Work out the finished part from the listing and answer in its coordinate system (mm). A direction names the side the tool comes from. Round coordinates to 2 decimals unless told otherwise and drop trailing zeros. Write each loop counter-clockwise with the first axis right and the second up, starting at its lowest first coordinate (ties: lowest second). Pieces come first, ordered by that corner, then holes.
from build123d import *

# Parameters (mm, degrees)
SKETCH2_W           = 20
SKETCH2_H           = 20
BOSS_EXTRUDE1_DEPTH = 25
SKETCH4_W           = 20
SKETCH4_H           = 20
BOSS_EXTRUDE2_DEPTH = 25
SKETCH5_R           = 6.5
BOSS_EXTRUDE3_DEPTH = 35
SKETCH7_R           = 6.5
BOSS_EXTRUDE4_DEPTH = 35
FILLET1_START       = -25
FILLET1_DEPTH       = 50
FILLET1_START_2     = 10
FILLET1_2_DEPTH     = 15
FILLET1_3_DEPTH     = 50
FILLET2_R           = 10
FILLET3_START       = -1e-07
FILLET3_DEPTH       = 25.0000001
FILLET3_START_2     = -25
FILLET3_2_DEPTH     = 34.870059035
FILLET3_START_3     = -10
FILLET3_3_DEPTH     = 20
FILLET4_R           = 10
FILLET5_START       = -25
FILLET5_DEPTH       = 50
FILLET5_2_DEPTH     = 24.9999999
FILLET5_START_2     = -10
FILLET5_3_DEPTH     = 20


with BuildPart() as part:
    # Sketch2 → Boss-Extrude1 (new, symmetric)
    with BuildSketch(Plane.XY):
        Rectangle(SKETCH2_W, SKETCH2_H)
    extrude(amount=BOSS_EXTRUDE1_DEPTH, both=True)

    # Sketch4 → Boss-Extrude2 (add, symmetric)
    with BuildSketch(Plane(origin=(0, 0, 0), x_dir=(1, 0, 0), z_dir=(0, 1, 0))):
        with Locations((10, 0)):
            Rectangle(SKETCH4_W, SKETCH4_H)
    extrude(amount=BOSS_EXTRUDE2_DEPTH, both=True)

    # Sketch5 → Boss-Extrude3 (add, symmetric)
    with BuildSketch(Plane(origin=(0, 0, 0), x_dir=(1, 0, 0), z_dir=(0, 1, 0))):
        with Locations(Location((10, 0, 0), (0, 0, 90))):
            Circle(SKETCH5_R)
    extrude(amount=BOSS_EXTRUDE3_DEPTH, both=True)

    # Sketch7 → Boss-Extrude4 (add, symmetric)
    with BuildSketch(Plane.XY):
        with Locations(Location((0, 0, 0), (0, 0, 180))):
            Circle(SKETCH7_R)
    extrude(amount=BOSS_EXTRUDE4_DEPTH, both=True)

    # Fillet1: read off the stored shape, not the designer's step
    # Fillet1 outline → Fillet1 (cut)
    with BuildSketch(Plane(origin=(0, 0, 0), x_dir=(1, 0, 0), z_dir=(0, 1, 0)).offset(FILLET1_START)):
        with BuildLine():
            Line((20, 10), (10, 10))
            ThreePointArc((10, 10), (17.071067812, 7.071067812), (20, 0))
            Line((20, 0), (20, 10))
        make_face()
    extrude(amount=FILLET1_DEPTH, mode=Mode.SUBTRACT)

    # Fillet1 2 outline → Fillet1 2 (cut)
    with BuildSketch(Plane(origin=(0, 0, 0), x_dir=(1, 0, 0), z_dir=(0, 1, 0)).offset(FILLET1_START_2)):
        with BuildLine():
            ThreePointArc((10, -10), (2.928932188, -7.071067812), (0, 0))
            Line((0, 0), (0, -10))
            Line((0, -10), (10, -10))
        make_face()
    extrude(amount=FILLET1_2_DEPTH, mode=Mode.SUBTRACT)

    # Fillet1 3 outline → Fillet1 3 (cut)
    with BuildSketch(Plane.XY.offset(FILLET1_START)):
        with BuildLine():
            Line((-10, 10), (-10, 0))
            ThreePointArc((-10, 0), (-7.071067812, 7.071067812), (0, 10))
            Line((0, 10), (-10, 10))
        make_face()
    extrude(amount=FILLET1_3_DEPTH, mode=Mode.SUBTRACT)

    # Fillet2
    fillet2_edges = [part.edges().sort_by_distance(p)[0] for p in [
        (20, 0, 10),
        (10, 10, -17.5),
        (10, -10, 17.5),
    ]]
    fillet(fillet2_edges, radius=FILLET2_R - 0.0001)  # a hair under: the kernel refuses the full size

    # Fillet3: read off the stored shape, not the designer's step
    # Fillet3 outline → Fillet3 (cut)
    with BuildSketch(Plane.XY.offset(FILLET3_START)):
        with BuildLine():
            Line((10, 10), (0, 10))
            ThreePointArc((0, 10), (7.071067812, 7.071067812), (10, 0))
            Line((10, 0), (10, 10))
        make_face()
        with BuildLine():
            Line((-10, -10), (0, -10))
            ThreePointArc((0, -10), (-7.071067812, -7.071067812), (-10, 0))
            Line((-10, 0), (-10, -10))
        make_face()
    extrude(amount=FILLET3_DEPTH, mode=Mode.SUBTRACT)

    # Fillet3 2 outline → Fillet3 2 (cut)
    with BuildSketch(Plane.XY.offset(FILLET3_START_2)):
        with BuildLine():
            Line((-10, -10), (0, -10))
            ThreePointArc((0, -10), (-7.071067812, -7.071067812), (-10, 0))
            Line((-10, 0), (-10, -10))
        make_face()
    extrude(amount=FILLET3_2_DEPTH, mode=Mode.SUBTRACT)

    # Fillet3 3 outline → Fillet3 3 (add)
    with BuildSketch(Plane(origin=(0, 0, 0), x_dir=(1, 0, 0), z_dir=(0, 1, 0)).offset(FILLET3_START_3)):
        with BuildLine():
            ThreePointArc((0, 0), (2.928932188, -7.071067812), (10, -10))
            Line((10, -10), (10, 1e-07))
            Line((10, 1e-07), (0, 0))
        make_face()
    extrude(amount=FILLET3_3_DEPTH)

    # Fillet4
    fillet4_edges = [part.edges().sort_by_distance(p)[0] for p in [
        (10, -10, -17.5),
    ]]
    fillet(fillet4_edges, radius=FILLET4_R - 0.0001)  # a hair under: the kernel refuses the full size

    # Fillet5: read off the stored shape, not the designer's step
    # Fillet5 outline → Fillet5 (cut)
    with BuildSketch(Plane(origin=(0, 0, 0), x_dir=(1, 0, 0), z_dir=(0, 1, 0)).offset(FILLET5_START)):
        with BuildLine():
            Line((0, 10), (0, 0))
            ThreePointArc((0, 0), (2.928932188, 7.071067812), (10, 10))
            Line((10, 10), (0, 10))
        make_face()
    extrude(amount=FILLET5_DEPTH, mode=Mode.SUBTRACT)

    # Fillet5 2 outline → Fillet5 2 (cut)
    with BuildSketch(Plane(origin=(0, 0, 0), x_dir=(1, 0, 0), z_dir=(0, 1, 0)).offset(FILLET5_START)):
        with BuildLine():
            ThreePointArc((10, -10), (2.928932188, -7.071067812), (0, 0))
            Line((0, 0), (0, -10))
            Line((0, -10), (10, -10))
        make_face()
    extrude(amount=FILLET5_2_DEPTH, mode=Mode.SUBTRACT)

    # Fillet5 3 outline → Fillet5 3 (add)
    with BuildSketch(Plane.XY.offset(FILLET5_START_2)):
        with BuildLine():
            ThreePointArc((10, 0), (7.071067812, 7.071067812), (0, 10))
            Line((0, 10), (0, -10))
            ThreePointArc((0, -10), (7.071067812, -7.071067812), (10, 0))
        make_face()
    extrude(amount=FILLET5_3_DEPTH)


solid = part.part
Q1. Given pin 1 (5 mm diameter, centred on x = -5.5, z = -3, fed in from -Y); pin 2 (8 mm diameter, centred on x = 2.5, z = -27.5, fed in from -Y); pin 3 (8 mm diameter, centred on y = 24.5, z = -15.5, fed in from -X); pin 4 (8 mm diameter, centred on y = 24, z = -6, fed in from +X), each flat-ended and moving along its own axis, determine where each tip first touches the part or whether it passes through.
Q2. Find the intervals of material crossed by L1, parallel to Z at x = -8, y = -5.5; L2, parallel to Y at x = 0.5, z = 9; L3, parallel to Z at x = 18.5, y = -17, in increasing order.
Q3. Find section D-D (x = 8). Determine the outline of the cut face in (y, z), plus the area to 3 significant figures.
Q4. A tool of negligible diameter and unlimited length cuts with its end or side. For faces 1 (the face through (7, 0, 25)), 2 (the face through (5.158, 3.955, -29.93)), 3 (the face through (6.99, -7.15, -17.4)), 4 (the face through (13.955, -29.93, 5.158)), from which of +Z, -Z, +X, -X, +Y, -Y can it reach the whole face along a straight path? Write none if from no direction.
Q5. Find section A-A (x = 15). Determine the outline of the cut face in (y, z), plus the area to 3 significant figures.
Report:
1. pin 1: stops at y = -9.54
1. pin 2: stops at y = -10
1. pin 3: passes through
1. pin 4: stops at x = 19.8
2. L1: z = -25 to 25
2. L2: y = -9.99 to 9.99
2. L3: z = -5.27 to 5.27
3. outline: (-35, -6.18) - (-25, -6.18) - (-25, -9.8) - (-6, -9.8) - (-6, -25) - (6, -25) - (6, -9.8) - (25, -9.8) - (25, -6.18) - (35, -6.18) - (35, 6.18) - (25, 6.18) - (25, 9.8) - (6, 9.8) - (6, 25) - (-6, 25) - (-6, 9.8) - (-25, 9.8) - (-25, 6.18) - (-35, 6.18) - close
3. area: 1,590 mm2
4. face 1: +Z
4. face 2: -Z
4. face 3: -Z, +X, -Y
4. face 4: -Y
5. outline: (-35, -4.15) - (-25, -4.15) - (-25, -8.66) - (25, -8.66) - (25, -4.15) - (35, -4.15) - (35, 4.15) - (25, 4.15) - (25, 8.66) - (-25, 8.66) - (-25, 4.15) - (-35, 4.15) - close
5. area: 1,030 mm2
